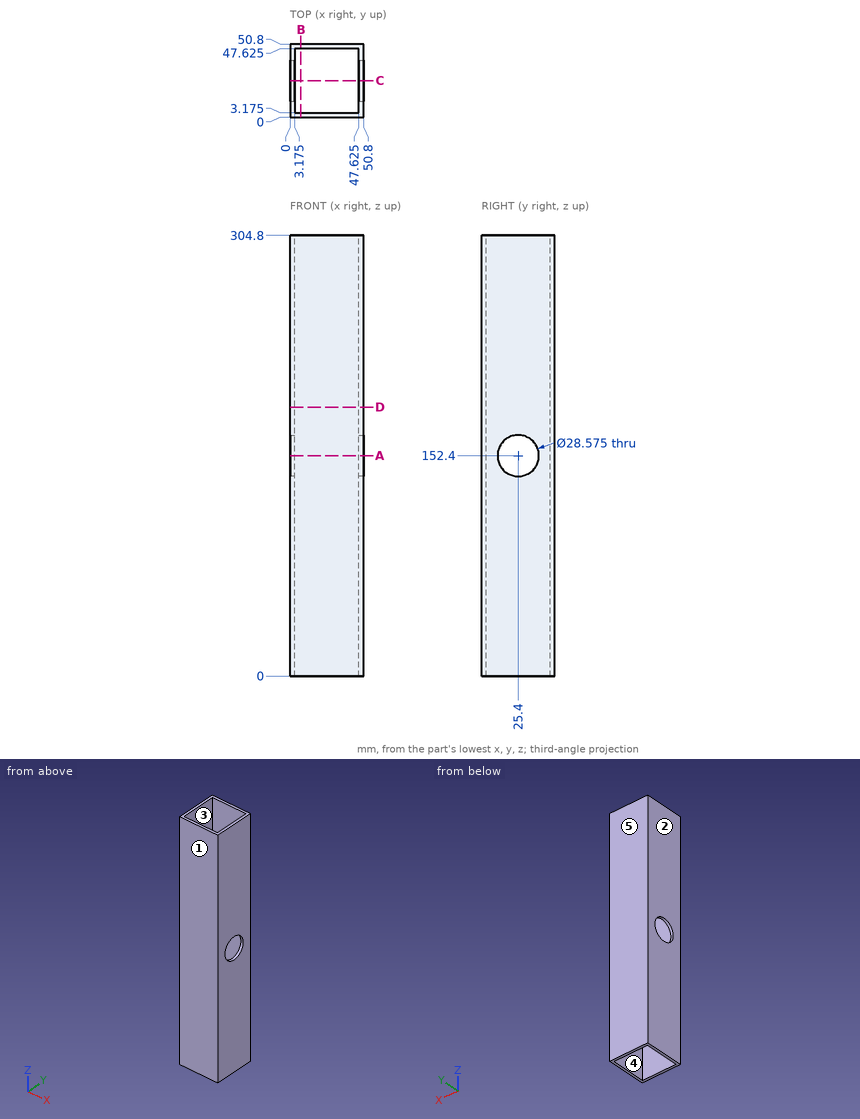
Here's the drawing with two shaded views (mm, measured from the low corner). I have some questions. A direction names the side the tool comes from. Give positions to 0.01 mm unless a question says otherwise; leave off trailing zeros. Order: outer loops, then holes, each group sorted by start corner. A loop starts at its lowest first (then second) coordinate and runs counter-clockwise, first axis right, second up. Notation, with made-up numbers: (-24.75, 86) - (20.25, 86) arc R18 cw to (20.25, 105) - close; hole circle Ø7 at (12.5, 41.25). An arc over 180 degrees is marked (long way). Use a Markdown table: item, result. Add a question column.
Q1. If we mould it in two halves opening along X, with no side actions, what happens to the marked faces 1, 2 and 3? For each: released by +X, released by -X, zero draft, split by the parting line, or undercut.
Q2. I'm going to push a flat-ended pin straight in: pin 1 (12 mm diameter, centred on x = 25, z = 227, fed in from -Y). Where does the tip first touch, or does it pass through?
Q3. If we section it at A-A on z = 152.4: Write out the boundary of the cut face in (x, y) (1 decimal), plus the area to 3 significant figures.
Q4. If we section it at B-B on x = 7.5: Write out the boundary of the cut face in (y, z) (3 decimals).
Q5. On a 3-axis mill with a long thin cutter (end or side, diameter ignored), from which of +Z, -Z, +X, -X, +Y, -Y can I reach the whole of each face in a straight line? I mean the marked faces 4 and 5. Say none if no direction works.
Q6. Please list where these lines run through material, in increasing order: line 1 along X through (y, z) = (13.5, 138.5) (3 decimals); line 2 along Z through (x, y) = (49, 25).
Q7. If we section it at D-D on z = 186: Write out the boundary of the cut face in (x, y) (3 decimals).
Q8. If we section it at C-C on y = 25.4: Write out the boundary of the cut face in (x, z) (1 decimal), plus the area to 3 significant figures.
Answers follow:
| question | item | result |
|---|---|---|
| 1 | face 1 | zero draft |
| 1 | face 2 | released by -X |
| 1 | face 3 | undercut |
| 2 | pin 1 | stops at y = 0 |
| 3 | outline | (0, 0) - (50.8, 0) - (50.8, 11.1) - (47.6, 11.1) - (47.6, 3.2) - (3.2, 3.2) - (3.2, 11.1) - (0, 11.1) - close; (0, 39.7) - (3.2, 39.7) - (3.2, 47.6) - (47.6, 47.6) - (47.6, 39.7) - (50.8, 39.7) - (50.8, 50.8) - (0, 50.8) - close |
| 3 | area | 423 mm^2 |
| 4 | outline | (0, 0) - (3.175, 0) - (3.175, 304.8) - (0, 304.8) - close; (47.625, 0) - (50.8, 0) - (50.8, 304.8) - (47.625, 304.8) - close |
| 5 | face 4 | +Z, -Z |
| 5 | face 5 | +Z, -Z, +X, -X, +Y |
| 6 | line 1 | x = 0 to 3.175, 47.625 to 50.8 |
| 6 | line 2 | z = 0 to 138.12, 166.68 to 304.8 |
| 7 | outline | (0, 0) - (50.8, 0) - (50.8, 50.8) - (0, 50.8) - close; hole (3.175, 3.175) - (47.625, 3.175) - (47.625, 47.625) - (3.175, 47.625) - close |
| 8 | outline | (0, 0) - (3.2, 0) - (3.2, 138.1) - (0, 138.1) - close; (0, 166.7) - (3.2, 166.7) - (3.2, 304.8) - (0, 304.8) - close; (47.6, 0) - (50.8, 0) - (50.8, 138.1) - (47.6, 138.1) - close; (47.6, 166.7) - (50.8, 166.7) - (50.8, 304.8) - (47.6, 304.8) - close |
| 8 | area | 1,750 mm^2 |
